from build123d import *

# Parameters (mm, degrees)
BOSS_EXTRUDE1_DEPTH = 41.3
SKETCH2_R           = 16
CUT_EXTRUDE2_DEPTH  = 41.3
CUT_EXTRUDE7_DEPTH  = 41.3
SKETCH8_R           = 1.6
CUT_EXTRUDE8_DEPTH  = 41.3
FILLET1_R           = 3


with BuildPart() as part:
    # Sketch1 → Boss-Extrude1 (new body)
    with BuildSketch(Plane(origin=(0, 0, 0), x_dir=(0, 0, -1), z_dir=(1, 0, 0))):
        Polygon((-1.5, -22.5), (-49.5, -22.5), (-49.5, -25.5), (1.5, -25.5), (1.5, -22.5), (1.5, 25.5), (-1.5, 25.5), align=None)
    extrude(amount=BOSS_EXTRUDE1_DEPTH)

    # Sketch2 → Cut-Extrude2 (cut)
    with BuildSketch(Plane.XY.offset(1.5)):
        with Locations((20.65, 1.5)):
            Circle(SKETCH2_R)
    extrude(amount=-CUT_EXTRUDE2_DEPTH, mode=Mode.SUBTRACT)

    # Sketch4 → Cut-Extrude7 (cut)
    with BuildSketch(Plane(origin=(0, 0, -1.5), x_dir=(-1, 0, 0), z_dir=(0, 0, -1))):
        with BuildLine():
            Line((-3.557549808, 20.356030754), (-3.550011366, 18.356044961))
            ThreePointArc((-3.550011366, 18.356044961), (-5.143969246, 16.750025573), (-6.749988634, 18.343983453))
            Line((-6.749988634, 18.343983453), (-6.757527076, 20.343969246))
            ThreePointArc((-6.757527076, 20.343969246), (-5.163569196, 21.949988634), (-3.557549808, 20.356030754))
        make_face()
        with BuildLine():
            Line((-34.55, 20.35), (-34.55, 18.35))
            ThreePointArc((-34.55, 18.35), (-36.15, 16.75), (-37.75, 18.35))
            Line((-37.75, 18.35), (-37.75, 20.35))
            ThreePointArc((-37.75, 20.35), (-36.15, 21.95), (-34.55, 20.35))
        make_face()
        with BuildLine():
            Line((-3.55, -10.65), (-3.55, -12.65))
            ThreePointArc((-3.55, -12.65), (-5.15, -14.25), (-6.75, -12.65))
            Line((-6.75, -12.65), (-6.75, -10.65))
            ThreePointArc((-6.75, -10.65), (-5.15, -9.05), (-3.55, -10.65))
        make_face()
        with BuildLine():
            Line((-34.55, -10.65), (-34.55, -12.65))
            ThreePointArc((-34.55, -12.65), (-36.15, -14.25), (-37.75, -12.65))
            Line((-37.75, -12.65), (-37.75, -10.65))
            ThreePointArc((-37.75, -10.65), (-36.15, -9.05), (-34.55, -10.65))
        make_face()
    extrude(amount=-CUT_EXTRUDE7_DEPTH, mode=Mode.SUBTRACT)

    # Sketch8 → Cut-Extrude8 (cut)
    with BuildSketch(Plane.XZ.offset(25.5)):
        with Locations((20.65, 44.35)):
            Circle(SKETCH8_R)
        with Locations((20.65, 13.35)):
            Circle(SKETCH8_R)
        with Locations((20.65, 28.85)):
            Circle(SKETCH8_R)
        with BuildLine():
            Line((37.75, 44.35), (37.75, 13.35))
            ThreePointArc((37.75, 13.35), (36.15, 11.75), (34.55, 13.35))
            Line((34.55, 13.35), (34.55, 44.35))
            ThreePointArc((34.55, 44.35), (36.15, 45.95), (37.75, 44.35))
        make_face()
        with BuildLine():
            Line((6.75, 44.35), (6.75, 13.35))
            ThreePointArc((6.75, 13.35), (5.15, 11.75), (3.55, 13.35))
            Line((3.55, 13.35), (3.55, 44.35))
            ThreePointArc((3.55, 44.35), (5.15, 45.95), (6.75, 44.35))
        make_face()
    extrude(amount=-CUT_EXTRUDE8_DEPTH, mode=Mode.SUBTRACT)

    # Fillet1
    fillet1_edges = [part.edges().sort_by_distance(p)[0] for p in [
        (41.3, 25.5, 0),
        (41.3, -24, 49.5),
        (0, -24, 49.5),
        (0, 25.5, 0),
    ]]
    fillet(fillet1_edges, radius=FILLET1_R)


solid = part.part
Geometry: final body of the model. Coordinates: model frame, mm. A direction names the side the tool comes from. Give positions to 0.01 mm unless a question says otherwise; leave off trailing zeros. Write each loop counter-clockwise with the first axis right and the second up, starting at its lowest first coordinate (ties: lowest second). Pieces come first, ordered by that corner, then holes. Notation, with made-up numbers: M 32.25,25 L 53.25,25 A25 cw 53.25,50 Z; hole C 71,5 d1. An arc over 180 degrees is marked long. Answer in a Markdown table with one row per item. Add a question column.
(1) Reachability of faces 1 (the cylindrical face through (36.11, -14.25, -0.02)), 2 (the flat face through (3.55, -24, 29)), 3 (the cylindrical face through (0.86, -24.02, 48.6)) from +Z, -Z, +X, -X, +Y, -Y: full face, straight path, thin tool, end or side. Return the list, or none.
(2) Section A-A on x = 20.65. Return loops of the section in (y, z).
(3) Mould query, pull axis Y, two halves, no side actions, for faces 4 (the flat face through (20, -22.5, 25)), 5 (the cylindrical face through (5.19, -9.05, -0.02)), 6 (the cylindrical face through (21.51, -24.02, 30.2)). Classes: +Y half, -Y half, draft (parallel to the pull), parting line (faces both ways), or undercut.
(4) Section B-B on z = 21. Return loops of the section in (x, y).
(5) First-contact query: pin 1 (20.5 mm diameter, centred on x = 27.5, z = 32, fed in from +Y); pin 2 (20.5 mm diameter, centred on x = 30.5, y = -10, fed in from +Z). Flat tips, straight axial feed; report the tip coordinate or a pass-through.
(6) Ray query, line 1 (Z direction, x = 20.65, y = -24.9); line 2 (Y direction, x = 20.65, z = 0); line 3 (X direction, y = -23, z = 13). Return the intervals inside material, ascending.
(7) Section D-D on x = 32.5. Return loops of the section in (y, z), and give its area (3 significant figures).
(8) Section C-C on y = -2. Return loops of the section in (x, z).
Result set:
| question | item | result |
|---|---|---|
| 1 | face 1 | +Z, -Z |
| 1 | face 2 | +Y, -Y |
| 1 | face 3 | +Z, -X, +Y, -Y |
| 2 | outline | M -25.5,-1.5 L -14.5,-1.5 L -14.5,1.5 L -22.5,1.5 L -22.5,11.75 L -25.5,11.75 Z; M -25.5,14.95 L -22.5,14.95 L -22.5,27.25 L -25.5,27.25 Z; M -25.5,30.45 L -22.5,30.45 L -22.5,42.75 L -25.5,42.75 Z; M -25.5,45.95 L -22.5,45.95 L -22.5,49.5 L -25.5,49.5 Z; M 17.5,-1.5 L 25.5,-1.5 L 25.5,1.5 L 17.5,1.5 Z |
| 3 | face 4 | +Y half |
| 3 | face 5 | undercut |
| 3 | face 6 | draft |
| 4 | outline | M 0,-25.5 L 3.55,-25.5 L 3.55,-22.5 L 0,-22.5 Z; M 6.75,-25.5 L 34.55,-25.5 L 34.55,-22.5 L 6.75,-22.5 Z; M 37.75,-25.5 L 41.3,-25.5 L 41.3,-22.5 L 37.75,-22.5 Z |
| 5 | pin 1 | stops at y = -22.5 |
| 5 | pin 2 | stops at z = 1.5 |
| 6 | line 1 | z = -1.5 to 11.75, 14.95 to 27.25, 30.45 to 42.75, 45.95 to 49.5 |
| 6 | line 2 | y = -25.5 to -14.5, 17.5 to 25.5 |
| 6 | line 3 | x = 0 to 3.59, 6.71 to 19.09, 22.21 to 34.59, 37.71 to 41.3 |
| 7 | outline | M -25.5,-1.5 L -9.25,-1.5 L -9.25,1.5 L -22.5,1.5 L -22.5,49.5 L -25.5,49.5 Z; M 12.25,-1.5 L 25.5,-1.5 L 25.5,1.5 L 12.25,1.5 Z |
| 7 | area | 232 mm^2 |
| 8 | outline | M 0,-1.5 L 5.04,-1.5 L 5.04,1.5 L 0,1.5 Z; M 36.26,-1.5 L 41.3,-1.5 L 41.3,1.5 L 36.26,1.5 Z |
